Geometry: final body of the model. Coordinates: model frame, mm. Give positions to 0.01 mm unless a question says otherwise; leave off trailing zeros. Order: outer loops, then holes, each group sorted by start corner. A loop starts at its lowest first (then second) coordinate and runs counter-clockwise, first axis right, second up. Notation, with made-up numbers: (-20, -31) - (8, -31) arc R33 cw to (8, 0) - close; hole circle Ø6 at (21.25, 77). An arc over 180 degrees is marked (long way). Use one line per item in the form item = value.
from build123d import *

# Parameters (mm, degrees)
F0_R     = 1.5875
F1_DEPTH = 3.3782
F2_D     = 19.05
F3_D     = 12.7
F4_DEPTH = 3.175


# Not quite as in the source:
# - a feature names something its author has since deleted; it is built from what else it names


with BuildPart() as f1:
    # F0 (on Top) → F1 (new body)
    with BuildSketch(Plane.XY):
        Polygon((38.1, 38.1), (-38.1, 38.1), (-38.1, -38.1), (0, -38.1), (38.1, -38.1), (38.1, 0), align=None)
        with Locations((-23.3484897763, 13.2784806192)):
            Circle(F0_R, mode=Mode.SUBTRACT)
    extrude(amount=F1_DEPTH)

    # F2 (through all)
    with Locations(Plane(origin=(0, 0, 0), x_dir=(1, 0, 0), z_dir=(0, 0, -1))):
        with Locations((19.05, -19.05), (19.05, 19.05), (-19.05, 19.05)):
            Hole(F2_D / 2)

    # F3 (through all)
    with Locations(Plane(origin=(0, 0, 0), x_dir=(1, 0, 0), z_dir=(0, 0, -1))):
        with Locations((0, 0)):
            Hole(F3_D / 2)

    # F0 (on Top) → F4 (join, symmetric)
    with BuildSketch(Plane.XY):
        with Locations((-23.3484897763, 13.2784806192)):
            Circle(F0_R)
    extrude(amount=F4_DEPTH, both=True)


solid = f1.part
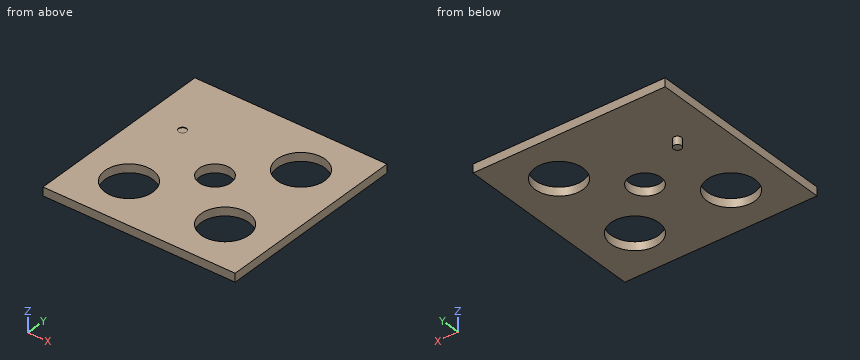
(1) Cut plane A-A on x = 0. Output: boundary loops of the cut face in (y, z), plus the area to 3 significant figures.
Computed values:
outline = (-38.1, 0) - (-6.35, 0) - (-6.35, 3.38) - (-38.1, 3.38) - close; (6.35, 0) - (38.1, 0) - (38.1, 3.38) - (6.35, 3.38) - close
area = 215 mm²
(2) Ray query, line 1 along Y through (x, z) = (19.05, 1.1) (3 decimals); line 2 along Y through (x, z) = (-5.5, 1.5); line 3 along Z through (x, y) = (-28.5, -8). Return the intervals inside material, ascending.
Computed values:
line_1 = -38.1 to -28.575, -9.525 to 9.525, 28.575 to 38.1
line_2 = -38.1 to -3.17, 3.17 to 38.1
line_3 = 0 to 3.38
(3) Contact query for flat-ended pins moving along their axis: pin 1 Ø16.5 at (x, y) = (0, 0) entering from -Z; pin 2 Ø3 at (y, z) = (-17, -1) entering from +X; pin 3 Ø1.5 at (y, z) = (26.5, -1.5) entering from -X; pin 4 Ø1.6 at (x, y) = (-23.5, 14) entering from +Z (3 decimals). Output: stop coordinate, or through.
Computed values:
pin_1 = 0
pin_2 = 38.1
pin_3 = through
pin_4 = 3.175
(4) Cut plane D-D on z = -1.5. Output: boundary loops of the cut face in (x, y) (1 decimal).
Computed values:
outline = circle Ø3.2 at (-23.3, 13.3)
(5) Cut plane C-C on x = 19.05. Output: boundary loops of the cut face in (y, z) (3 decimals).
Computed values:
outline = (-38.1, 0) - (-28.575, 0) - (-28.575, 3.378) - (-38.1, 3.378) - close; (-9.525, 0) - (9.525, 0) - (9.525, 3.378) - (-9.525, 3.378) - close; (28.575, 0) - (38.1, 0) - (38.1, 3.378) - (28.575, 3.378) - close
